Autodesk Inventor part; units mm, degrees
ref_plane "YZ Plane" through (0, 0, 0) normal (1, 0, 0) x (0, 1, 0)
ref_plane "XZ Plane" through (0, 0, 0) normal (0, 1, 0) x (-1, 0, 0)
ref_plane "XY Plane" through (0, 0, 0) normal (0, 0, 1) x (1, 0, 0)
sketch "スケッチ1" plane through (0, 0, 0) normal (0, 0, 1) x (1, 0, 0)
  circle A0 centre (0, 0) radius 1.5
  dimension "d0" = 3
extrude "押し出し1" add sketch "スケッチ1" along normal blind 6
sketch "スケッチ2" plane through (0, 0, 6) normal (0, 0, 1) x (1, 0, 0)
  circle A0 centre (0, 0) radius 1.5
  circle A1 centre (0, 0) radius 3
  dimension "d3" = 6
extrude "押し出し2" add sketch "スケッチ2" along normal blind 2 contours A0 | A1
fillet "フィレット1" radius 2 1 edges at (-3, 0, 8)
thread "ねじ1"
sketch "スケッチ3" plane through (0, 0, 0) normal (0, 0, -1) x (-1, 0, 0)
  circle A0 centre (0, 0) radius 1.5
extrude "押し出し3" add sketch "スケッチ3" along normal blind 9
sketch "スケッチ4" plane through (0, 0, -9) normal (0, 0, -1) x (-1, 0, 0)
  circle A0 centre (0, 0) radius 1.5
extrude "押し出し4" add sketch "スケッチ4" along normal blind 25
properties part number "SB　40mmなべネジ" material "Steel, Mild"
Verification items for the finished model (mm, model axes). A direction names the side the tool comes from. Give positions to 0.01 mm unless a question says otherwise; leave off trailing zeros. Write each loop counter-clockwise with the first axis right and the second up, starting at its lowest first coordinate (ties: lowest second). Pieces come first, ordered by that corner, then holes. Notation, with made-up numbers: M 15.5,73.5 L 44.5,73.5 A14 cw 44.5,93.5 Z; hole C 54,-25.5 d9. An arc over 180 degrees is marked long. Put each result on its own line as item: value. Start each with the question number.
1. Section check A-A (z = -3). Record the cut outline in (x, y).
2. Scan lines: line 1 along Y through (x, z) = (0, 2); line 2 along Z through (x, y) = (-1.5, 1.5); line 3 along X through (y, z) = (0.25, -17). Record each from-to range of solid material in increasing order. Write a range as [from, to].
3. Set-up check for faces 1 (the face through (0, 0, 8)), 2 (the face through (1.3, -1.3, 6)): record each of +Z, -Z, +X, -X, +Y, -Y from which the full face is reachable in a straight line by a thin tool's end or side.
4. Go/stop test with flat-tipped pins: pin 1 Ø1.5 at (x, z) = (0, 1.5) entering from -Y; pin 2 Ø1.5 at (x, z) = (1, -3.5) entering from +Y; pin 3 Ø1 at (y, z) = (-1, -19.5) entering from -X. Record where each tip stops, or that it passes through.
Answer list:
1. outline: C 0,0 d3
2. line 1: [-1.5, 1.5]
2. line 2: [6, 7.66]
2. line 3: [-1.48, 1.48]
3. face 1: +Z, +X, -X, +Y, -Y
3. face 2: -Z
4. pin 1: y = -1.5
4. pin 2: y = 1.48
4. pin 3: x = -1.41
